Answer from the drawing. Dimensions are ordinates in mm from the lowest x, y and z of the part. Round coordinates to 2 decimals unless told otherwise and drop trailing zeros. Order: outer loops, then holes, each group sorted by start corner. A loop starts at its lowest first (then second) coordinate and runs counter-clockwise, first axis right, second up. Notation, with made-up numbers: (-14.5, 22.5) -> (13.5, 22.5) arc R20 cw to (13.5, 60.5) -> close; hole circle Ø2 at (-38.75, 27). An arc over 180 degrees is marked (long way). Use a Markdown table: item, result. Add a question column.
Item 1: Find the intervals of material crossed by L1, parallel to X at y = 22, z = 2; L2, parallel to Y at x = 21, z = 0.65; L3, parallel to Z at x = 20, y = 13, in increasing order. Write a range as [from, to].
Item 2: A cutting plane is placed at D-D, the plane x = 8.25. Determine the outline of the cut face in (y, z).
Item 3: For a pull along Y with two mould halves and no side action, classify the marked faces 1, 2 and 3 as +Y half, -Y half, draft (parallel to the pull), parting line (faces both ways), or undercut.
Item 4: A cutting plane is placed at B-B, the plane x = 21. Determine the outline of the cut face in (y, z).
Item 5: A cutting plane is placed at C-C, the plane z = 1.4. Determine the outline of the cut face in (x, y).
Item 6: Flat-ended cylindrical pins translate along their axes: P1, Ø3, axis at x = 11, y = 22, coming from the -Z side; P2, Ø5, axis at x = 21, y = 12, coming from the +Z side; P3, Ø3, axis at y = 13, z = 3, coming from the -X side. Find the tip coordinate at first contact, or state that the pin passes through.
Item 7: A cutting plane is placed at A-A, the plane y = 22. Determine the outline of the cut face in (x, z).
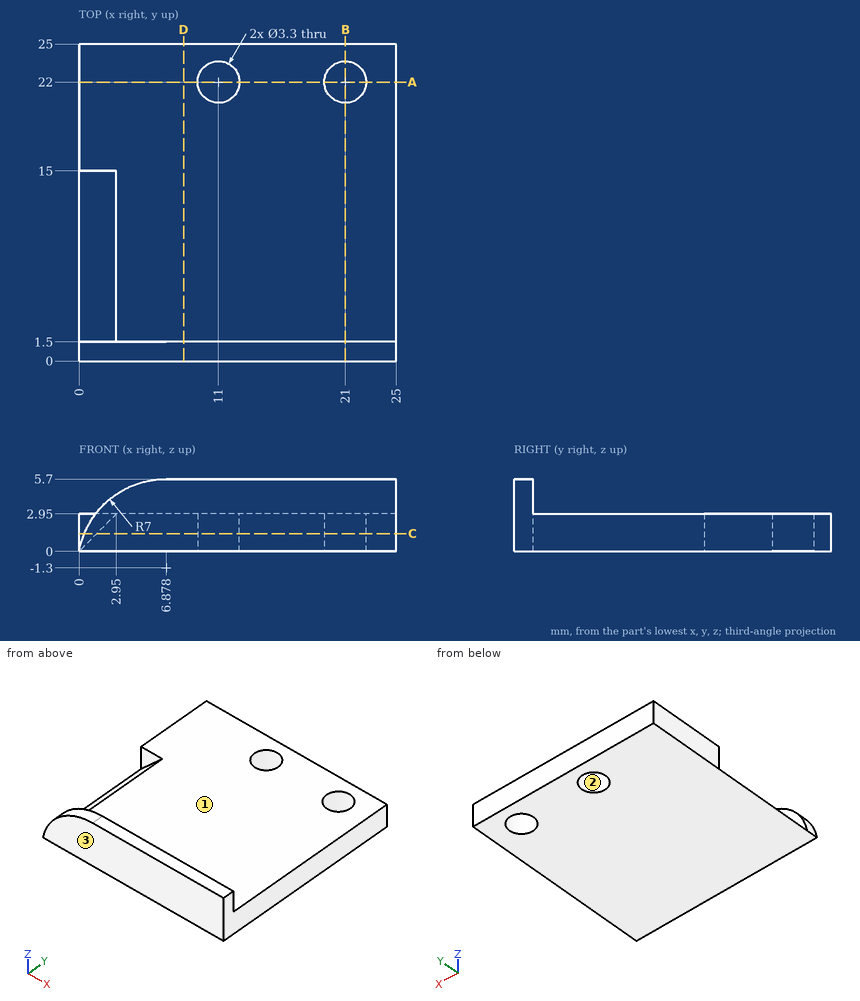
Reported:
| question | item | result |
|---|---|---|
| 1 | L1 | [0, 9.35], [12.65, 19.35], [22.65, 25] |
| 1 | L2 | [0, 20.35], [23.65, 25] |
| 1 | L3 | [0, 2.95] |
| 2 | outline | (0, 0) -> (25, 0) -> (25, 2.95) -> (1.5, 2.95) -> (1.5, 5.7) -> (0, 5.7) -> close |
| 3 | face 1 | draft |
| 3 | face 2 | undercut |
| 3 | face 3 | -Y half |
| 4 | outline | (0, 0) -> (20.35, 0) -> (20.35, 2.95) -> (1.5, 2.95) -> (1.5, 5.7) -> (0, 5.7) -> close; (23.65, 0) -> (25, 0) -> (25, 2.95) -> (23.65, 2.95) -> close |
| 5 | outline | (0, 15) -> (1.4, 15) -> (1.4, 1.5) -> (0.42, 1.5) -> (0.42, 0) -> (25, 0) -> (25, 25) -> (0, 25) -> close; hole circle Ø3.3 at (11, 22); hole circle Ø3.3 at (21, 22) |
| 6 | P1 | through |
| 6 | P2 | z = 2.95 |
| 6 | P3 | x = 1.5 |
| 7 | outline | (0, 0) -> (9.35, 0) -> (9.35, 2.95) -> (0, 2.95) -> close; (12.65, 0) -> (19.35, 0) -> (19.35, 2.95) -> (12.65, 2.95) -> close; (22.65, 0) -> (25, 0) -> (25, 2.95) -> (22.65, 2.95) -> close |
